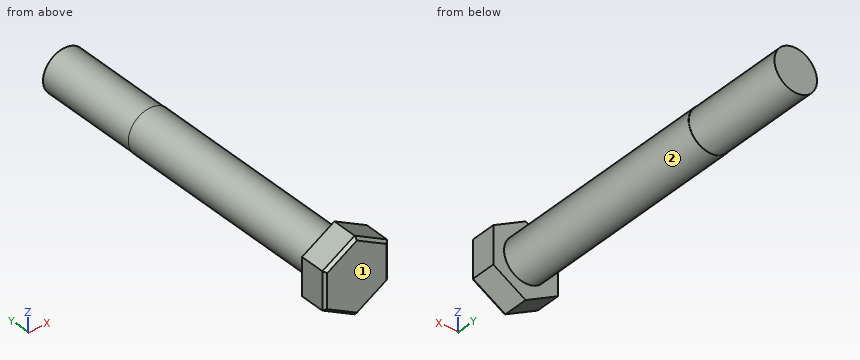
from build123d import *

# Parameters (mm, degrees)
F1_DEPTH = 10
F2_SIZE2 = 1
F2_SIZE  = 1
F3_R     = 8
F4_DEPTH = 120
F5_R     = 8
F5_R_2   = 7.9
F6_DEPTH = 38


with BuildPart() as f1:
    # F0 (on Front) → F1 (new body)
    with BuildSketch(Plane.XZ):
        Polygon((0, -13.856406), (12, -6.928203), (12, 6.928203), (0, 13.856406), (-12, 6.928203), (-12, -6.928203), align=None)
    extrude(amount=F1_DEPTH)

    # F2
    f2_edges = [f1.edges().sort_by_distance(p)[0] for p in [
        (6, -10, 10.392305),
        (-6, -10, 10.392305),
        (12, -10, 0),
        (6, -10, -10.392305),
        (-6, -10, -10.392305),
        (-12, -10, 0),
    ]]
    chamfer(f2_edges, length=F2_SIZE, length2=F2_SIZE2)

    # F3 (on face) → F4 (join)
    with BuildSketch(Plane(origin=(0, 0, 0), x_dir=(-1, 0, 0), z_dir=(0, 1, 0))):
        Circle(F3_R)
    extrude(amount=F4_DEPTH)

    # F5 (on face) → F6 (cut)
    with BuildSketch(Plane(origin=(0, 120, 0), x_dir=(-1, 0, 0), z_dir=(0, 1, 0))):
        Circle(F5_R)
        Circle(F5_R_2, mode=Mode.SUBTRACT)
    extrude(amount=-F6_DEPTH, mode=Mode.SUBTRACT)


solid = f1.part
Check sheet for the modelled part. Datum: model origin and axes. Units: mm. Face numbers are marked on the shaded views. A direction names the side the tool comes from. Coordinates: 2 decimals unless noted, no trailing zeros. Loops run counter-clockwise (first coordinate to the right, second up) from the corner with the lowest first, then second, coordinate; pieces in that order, holes last. Notation, with made-up numbers: (50, 67) -> (95, 67) arc R18 ccw to (95, 72) -> close; hole circle Ø8 at (-39.75, 32.25). An arc over 180 degrees is marked (long way). Answer in a Markdown table with one row per item.
1. Sectioned sample at D-D, the plane z = 10. Record the boundary of the cut face in (x, y), then the cut area to 3 significant figures.
Check values:
| item | result |
|---|---|
| outline | (-6.68, -9) -> (-4.68, -10) -> (4.68, -10) -> (6.68, -9) -> (6.68, 0) -> (-6.68, 0) -> close |
| area | 132 mm2 |
2. Material ranges on line 1 along X through (y, z) = (86, -0.25); line 2 along Y through (x, z) = (-9, 3.75); line 3 along Z through (x, y) = (-0.25, 49.5), recorded low to high. Write a range as [from, to].
Check values:
| item | result |
|---|---|
| line 1 | x = [-7.9, 7.9] |
| line 2 | y = [-10, 0] |
| line 3 | z = [-8, 8] |
3. Access from +Z, -Z, +X, -X, +Y, -Y to the whole of each face (thin tool, end or side, straight path). Record for the marked faces 1 and 2.
Check values:
| item | result |
|---|---|
| face 1 | +Z, -Z, +X, -X, -Y |
| face 2 | +Y |
4. Go/stop test with flat-tipped pins: pin 1 (8 mm diameter, centred on x = -4, y = 51, fed in from -Z); pin 2 (1 mm diameter, centred on x = 0, y = 5, fed in from +Z); pin 3 (6 mm diameter, centred on y = 10, z = 7, fed in from +X). Record where each tip stops, or that it passes through.
Check values:
| item | result |
|---|---|
| pin 1 | stops at z = -8 |
| pin 2 | stops at z = 8 |
| pin 3 | stops at x = 6.93 |
5. Sectioned sample at C-C, the plane y = 96. Record the boundary of the cut face in (x, z).
Check values:
| item | result |
|---|---|
| outline | circle Ø15.8 at (0, 0) |
6. Sectioned sample at A-A, the plane z = 0. Record the boundary of the cut face in (x, y).
Check values:
| item | result |
|---|---|
| outline | (-12, -9) -> (-11, -10) -> (11, -10) -> (12, -9) -> (12, 0) -> (8, 0) -> (8, 82) -> (7.9, 82) -> (7.9, 120) -> (-7.9, 120) -> (-7.9, 82) -> (-8, 82) -> (-8, 0) -> (-12, 0) -> close |
7. Sectioned sample at B-B, the plane x = 5.5. Record the boundary of the cut face in (y, z), then the cut area to 3 significant figures.
Check values:
| item | result |
|---|---|
| outline | (-10, -9.53) -> (-9, -10.68) -> (0, -10.68) -> (0, -5.81) -> (82, -5.81) -> (82, -5.67) -> (120, -5.67) -> (120, 5.67) -> (82, 5.67) -> (82, 5.81) -> (0, 5.81) -> (0, 10.68) -> (-9, 10.68) -> (-10, 9.53) -> close |
| area | 1,600 mm2 |
